```python
from build123d import *

# Parameters (mm, degrees)
SKETCH_5_W          = 80
SKETCH_5_H          = 25
EXTRUDE_4_DEPTH     = 90
SKETCH_6_R          = 2
SKETCH_6_R_2        = 11
CUT_EXTRUDE_1_DEPTH = 90
SKETCH_6_3_R        = 27
SKETCH_6_3_R_2      = 2
SKETCH_6_3_R_3      = 11
CUT_EXTRUDE_2_DEPTH = 1.5


with BuildPart() as part:
    # 草图5 → 凸台-拉伸4 (new body)
    with BuildSketch(Plane(origin=(0, 0, 0), x_dir=(1, 0, 0), z_dir=(0, 1, 0))):
        Rectangle(SKETCH_5_W, SKETCH_5_H)
    extrude(amount=EXTRUDE_4_DEPTH)

    # 草图6 → 切除-拉伸1 (cut)
    with BuildSketch(Plane.XY.offset(12.5)):
        with Locations((-18, 60)):
            Circle(SKETCH_6_R)
        with Locations((0, 60)):
            Circle(SKETCH_6_R_2)
        with Locations((18, 60)):
            Circle(SKETCH_6_R)
    extrude(amount=-CUT_EXTRUDE_1_DEPTH, mode=Mode.SUBTRACT)

    # 草图6<3> → 切除-拉伸2 (cut)
    with BuildSketch(Plane.XY.offset(12.5)):
        with Locations((0, 60)):
            Circle(SKETCH_6_3_R)
        with Locations((-18, 60)):
            Circle(SKETCH_6_3_R_2, mode=Mode.SUBTRACT)
        with Locations((0, 60)):
            Circle(SKETCH_6_3_R_3, mode=Mode.SUBTRACT)
        with Locations((18, 60)):
            Circle(SKETCH_6_3_R_2, mode=Mode.SUBTRACT)
    extrude(amount=-CUT_EXTRUDE_2_DEPTH, mode=Mode.SUBTRACT)


solid = part.part
```
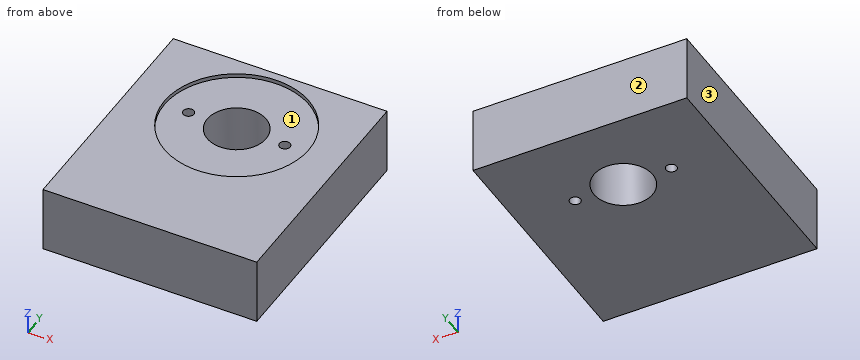
Part model, mm, in its own coordinate system. Face numbers are marked on the shaded views. Round coordinates to 2 decimals unless told otherwise and drop trailing zeros. Loops run counter-clockwise (first coordinate to the right, second up) from the corner with the lowest first, then second, coordinate; pieces in that order, holes last. Notation, with made-up numbers: (77, -5.5) -> (84, -5.5) arc R20 ccw to (84, 11.5) -> close; hole circle Ø2 at (44, 6.25). An arc over 180 degrees is marked (long way). Use a Markdown table: item, result.
1) Pull direction X, two halves, no side cores. Call the marked faces 1, 2 and 3: pulls with the +X half, pulls with the -X half, needs draft (parallel to the pull), parting line crosses it, or undercut.
The answers:
| item | result |
|---|---|
| face 1 | undercut |
| face 2 | needs draft |
| face 3 | pulls with the -X half |
2) Drop flat-ended pins along their axis: pin 1 Ø3.5 at (x, y) = (-18, 60) entering from -Z; pin 2 Ø8 at (x, y) = (22, 56) entering from +Z. Give the stop position or say it passes through.
The answers:
| item | result |
|---|---|
| pin 1 | passes through |
| pin 2 | stops at z = 11 |
3) Probe line 1 (Y direction, x = -18, z = -0.5); line 2 (Y direction, x = 0, z = -2.5); line 3 (Z direction, x = -6.5, y = 45.5). List the from-to ranges inside material, lowest first. Write a range as [from, to].
The answers:
| item | result |
|---|---|
| line 1 | y = [0, 58], [62, 90] |
| line 2 | y = [0, 49], [71, 90] |
| line 3 | z = [-12.5, 11] |
4) Cut at C-C, the plane z = 3.75. List the corners of the cut face in (x, y).
The answers:
| item | result |
|---|---|
| outline | (-40, 0) -> (40, 0) -> (40, 90) -> (-40, 90) -> close; hole circle Ø4 at (-18, 60); hole circle Ø22 at (0, 60); hole circle Ø4 at (18, 60) |
5) Cut at D-D, the plane y = 84. List the corners of the cut face in (x, z).
The answers:
| item | result |
|---|---|
| outline | (-40, -12.5) -> (40, -12.5) -> (40, 12.5) -> (12.37, 12.5) -> (12.37, 11) -> (-12.37, 11) -> (-12.37, 12.5) -> (-40, 12.5) -> close |
6) Cut at A-A, the plane y = 60. List the corners of the cut face in (x, z).
The answers:
| item | result |
|---|---|
| outline | (-40, -12.5) -> (-20, -12.5) -> (-20, 11) -> (-27, 11) -> (-27, 12.5) -> (-40, 12.5) -> close; (-16, -12.5) -> (-11, -12.5) -> (-11, 11) -> (-16, 11) -> close; (11, -12.5) -> (16, -12.5) -> (16, 11) -> (11, 11) -> close; (20, -12.5) -> (40, -12.5) -> (40, 12.5) -> (27, 12.5) -> (27, 11) -> (20, 11) -> close |
7) Cut at B-B, the plane x = 0. List the corners of the cut face in (y, z), and give its area (3 significant figures).
The answers:
| item | result |
|---|---|
| outline | (0, -12.5) -> (49, -12.5) -> (49, 11) -> (33, 11) -> (33, 12.5) -> (0, 12.5) -> close; (71, -12.5) -> (90, -12.5) -> (90, 12.5) -> (87, 12.5) -> (87, 11) -> (71, 11) -> close |
| area | 1,650 mm2 |
